Autodesk Inventor part; units mm, degrees
ref_plane "YZ Plane" through (0, 0, 0) normal (1, 0, 0) x (0, 1, 0)
ref_plane "XZ Plane" through (0, 0, 0) normal (0, 1, 0) x (-1, 0, 0)
ref_plane "XY Plane" through (0, 0, 0) normal (0, 0, 1) x (1, 0, 0)
sketch "Sketch1" plane through (0, 0, 0) normal (0, 0, 1) x (1, 0, 0)
  line L0 (21.844, 0) -> (21.844, -12.7)
  line L1 (25.019, -15.875) -> (38.1, -15.875)
  line L2 (38.1, -15.875) -> (38.1, -18.415)
  line L3 (38.1, -18.415) -> (19.304, -18.415)
  line L4 (19.304, -18.415) -> (19.304, 0)
  line L5 (19.304, 0) -> (21.844, 0)
  line L6 (0, 0) -> (27.9096, 0) construction
  arc A0 (21.844, -12.7) -> (25.019, -15.875) centre (25.019, -12.7) ccw
  line L7 (0, 0) -> (0, -18.415) construction
  dimension "d0" = 19.304
  dimension "d1" = 18.415
  dimension "d2" = 2.54
  dimension "d3" = 2.54
  dimension "d5" = 3.175
  dimension "d9" = 38.1
revolve "Revolution1" add sketch "Sketch1" angle 360 about axis through (0, 0, 0) along (0, -1, 0)
sketch "Sketch2" plane through (0, 0, 0) normal (1, 0, 0) x (0, 1, 0)
  line L0 (0, 0) -> (-26.67, 0) construction
  line L1 (-13.97, -6.35) -> (0, -6.35)
  line L2 (0, -6.35) -> (0, 6.35)
  line L3 (0, 6.35) -> (-13.97, 6.35)
  line L4 (-13.97, 6.35) -> (-13.97, -6.35)
  line L5 (-13.97, -6.35) -> (0, 6.35) construction
  line L6 (0, -6.35) -> (-13.97, 6.35) construction
  line L7 (0, 19.304) -> (0, -19.304)
  point P0 (-6.985, 0)
  dimension "d10" = 12.7
  dimension "d11" = 13.97
  dimension "d12" = 0
extrude "Extrusion1" cut sketch "Sketch2" along normal blind 22.86
properties part number "customWasher"
Check sheet for the modelled part. Datum: model origin and axes. Units: mm. A direction names the side the tool comes from. Give positions to 0.01 mm unless a question says otherwise; leave off trailing zeros. Order: outer loops, then holes, each group sorted by start corner. A loop starts at its lowest first (then second) coordinate and runs counter-clockwise, first axis right, second up. Notation, with made-up numbers: M 34,40 L 81,40 A29 ccw 81,63 Z; hole C 5,55.5 d8. An arc over 180 degrees is marked long. Answer in a Markdown table with one row per item.
1) Release check for a two-part mould opening along X. For faces 1 (the flat face through (-9, -18.415, 17.5)), 2 (the cylindrical face through (-30.235, -17.163, -23.183)), 3 (the cylindrical face through (-19.285, -9.079, -0.849)) record: +X half, -X half, draft (parallel to the pull), parting line (faces both ways), or undercut.
Filled sheet:
| item | result |
|---|---|
| face 1 | draft |
| face 2 | parting line |
| face 3 | undercut |
2) Cross-section at B-B, the plane x = 0. Enter the section's corners in (y, z) (3 decimals).
Filled sheet:
| item | result |
|---|---|
| outline | M -18.415,-38.1 L -15.875,-38.1 L -15.875,-25.019 A3.175 cw -12.7,-21.844 L 0,-21.844 L 0,-19.304 L -18.415,-19.304 Z; M -18.415,19.304 L 0,19.304 L 0,21.844 L -12.7,21.844 A3.175 cw -15.875,25.019 L -15.875,38.1 L -18.415,38.1 Z |
3) Gauge pin test, flat ends, axial feed: P1, Ø8, axis at x = 16, y = -16, coming from the -Z side; P2, Ø1.9, axis at x = 19.5, z = 2, coming from the +Y side; P3, Ø1, axis at x = 18, y = -15.5, coming from the -Z side. Record the tip position at first contact, or that the pin passes through.
Filled sheet:
| item | result |
|---|---|
| P1 | stops at z = -36.16 |
| P2 | stops at y = -13.97 |
| P3 | stops at z = -33.76 |
4) Cross-section at C-C, the plane y = -5. Enter the section's corners in (x, z).
Filled sheet:
| item | result |
|---|---|
| outline | M 18.23,-6.35 A19.3 cw long 18.23,6.35 L 20.9,6.35 A21.84 ccw long 20.9,-6.35 Z |
5) Thickness scan on L1, parallel to Z at x = 0, y = -4.5; L2, parallel to Y at x = -29.5, z = -6.5 (3 decimals); L3, parallel to Z at x = 0, y = -14.25. Record the ranges inside material, lowest first. Write a range as [from, to].
Filled sheet:
| item | result |
|---|---|
| L1 | z = [-21.84, -19.3], [19.3, 21.84] |
| L2 | y = [-18.415, -15.875] |
| L3 | z = [-22.25, -19.3], [19.3, 22.25] |
6) Access from +Z, -Z, +X, -X, +Y, -Y to the whole of each face (thin tool, end or side, straight path). Record for faces 4 (the flat face through (-20, 0, 0)), 5 (the flat face through (21, -13.97, 0)), 6 (the cylindrical face through (-21.827, -6.439, 0.87)).
Filled sheet:
| item | result |
|---|---|
| face 4 | +Z, -Z, +X, -X, +Y |
| face 5 | +X, +Y |
| face 6 | +Y |
7) Cross-section at A-A, the plane z = 0. Enter the section's corners in (x, y) (3 decimals).
Filled sheet:
| item | result |
|---|---|
| outline | M -38.1,-18.415 L -19.304,-18.415 L -19.304,0 L -21.844,0 L -21.844,-12.7 A3.175 cw -25.019,-15.875 L -38.1,-15.875 Z; M 19.304,-18.415 L 38.1,-18.415 L 38.1,-15.875 L 25.019,-15.875 A3.175 cw 22.109,-13.97 L 19.304,-13.97 Z |
